from build123d import *

# Parameters (mm, degrees)
BOSS_EXTRUDE1_DEPTH      = 25
BOSS_EXTRUDE1_DEPTH_BACK = 25
SKETCH2_R                = 1.75
CUT_EXTRUDE1_DEPTH       = 29.722813233
BOSS_EXTRUDE2_DEPTH      = 3


with BuildPart() as part:
    # Sketch1 → Boss-Extrude1 (new, two sides: drawn at the far end of the back side and taken through both)
    with BuildSketch(Plane.XY.offset(-BOSS_EXTRUDE1_DEPTH_BACK)):
        Polygon((-10, 0), (0, 0), (5.773502692, 10), (3.464101615, 10), (-1.154700538, 2), (-10, 2), align=None)
    extrude(amount=BOSS_EXTRUDE1_DEPTH + BOSS_EXTRUDE1_DEPTH_BACK)

    # Sketch2 → Cut-Extrude1 (cut, through all)
    with BuildSketch(Plane.XZ):
        with Locations(Location((-7, 17.5, 0), (0, 0, 270))):
            Circle(SKETCH2_R)
        with Locations(Location((-7, -17.5, 0), (0, 0, 270))):
            Circle(SKETCH2_R)
    extrude(amount=-CUT_EXTRUDE1_DEPTH, mode=Mode.SUBTRACT)

    # Sketch3 → Boss-Extrude2 (add)
    with BuildSketch(Plane(origin=(0, 0, -25), x_dir=(-1, 0, 0), z_dir=(0, 0, -1))):
        Polygon((-3.464101615, 10), (10, 2), (1.154700538, 2), align=None)
    boss_extrude2 = extrude(amount=-BOSS_EXTRUDE2_DEPTH)

    # Mirror1: Boss-Extrude2 across plane
    add(boss_extrude2.mirror(Plane.XY))


solid = part.part
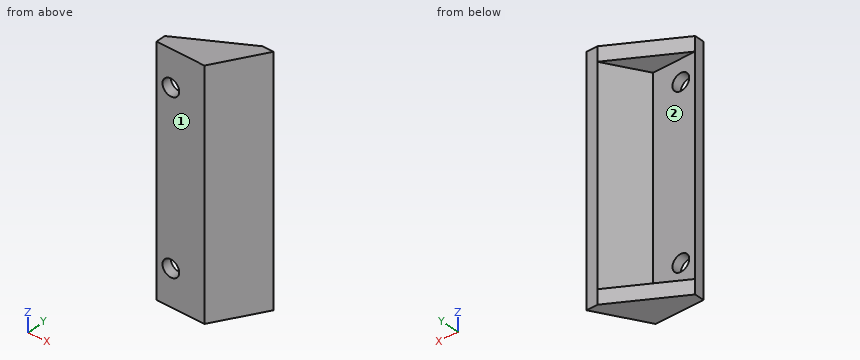
The listing builds one solid part. Answer for the finished solid, in the listing's coordinates (mm). Face numbers are marked on the shaded views. A direction names the side the tool comes from. Coordinates: 2 decimals unless noted, no trailing zeros. Loops run counter-clockwise (first coordinate to the right, second up) from the corner with the lowest first, then second, coordinate; pieces in that order, holes last. Notation, with made-up numbers: (-27.5, 2) -> (1.5, 2) arc R20 ccw to (1.5, 20) -> close; hole circle Ø9 at (-37.75, 16.5). An arc over 180 degrees is marked (long way). Write item = value, one per line. Start each with the question number.
1) A cutting plane is placed at C-C (z = -9.5). Give the vertices of the cut face in (x, y).
2) A tool of negligible diameter and unlimited length cuts with its end or side. For the marked faces 1 and 2, from which of +Z, -Z, +X, -X, +Y, -Y can it reach the whole face along a straight path? Write none if from no direction.
3) Given pin 1 Ø6 at (y, z) = (9, -2.5) entering from +X; pin 2 Ø3 at (x, z) = (-7, -17.5) entering from -Y; pin 3 Ø1 at (x, z) = (1.5, -17) entering from +Y; pin 4 Ø1.5 at (x, z) = (-0.5, 13) entering from +Y, each flat-ended and moving along its own axis, determine where each tip first touches the part or whether it passes through.
4) Straight lines are drawn through the part: line 1 (Z direction, x = -5, y = 3.5); line 2 (Y direction, x = -8.25, z = -5.5); line 3 (X direction, y = 1.65, z = -17.5). For each, find the intervals that lie inside material, in ascending order. Write a range as from..to.
5) A cutting plane is placed at A-A (x = -7). Give the vertices of the cut face in (y, z).
6) A cutting plane is placed at D-D (x = -3). Give the vertices of the cut face in (y, z).
7) A cutting plane is placed at B-B (z = -17.5). Give the vertices of the cut face in (x, y), then the cut area to 3 significant figures.
Responses:
q1.outline = (-10, 0) -> (0, 0) -> (5.77, 10) -> (3.46, 10) -> (-1.15, 2) -> (-10, 2) -> close
q2.face_1 = +Z, -Z, +X, -X, -Y
q2.face_2 = -X, +Y
q3.pin_1 = 5.77
q3.pin_2 = through
q3.pin_3 = 7.46
q3.pin_4 = 4.43
q4.line_1 = -25..-22, 22..25
q4.line_2 = 0..2
q4.line_3 = -10..-8.75, -5.25..0.95
q5.outline = (0, -25) -> (3.78, -25) -> (3.78, -22) -> (2, -22) -> (2, -19.25) -> (0, -19.25) -> close; (0, -15.75) -> (2, -15.75) -> (2, 15.75) -> (0, 15.75) -> close; (0, 19.25) -> (2, 19.25) -> (2, 22) -> (3.78, 22) -> (3.78, 25) -> (0, 25) -> close
q6.outline = (0, -25) -> (6.16, -25) -> (6.16, -22) -> (2, -22) -> (2, 22) -> (6.16, 22) -> (6.16, 25) -> (0, 25) -> close
q7.outline = (-10, 0) -> (-8.75, 0) -> (-8.75, 2) -> (-10, 2) -> close; (-5.25, 0) -> (0, 0) -> (5.77, 10) -> (3.46, 10) -> (-1.15, 2) -> (-5.25, 2) -> close
q7.area = 32.6 mm²
